```python
from build123d import *

# Parameters (mm, degrees)
BOSS_EXTRUDE1_DEPTH = 244.475
SKETCH2_R           = 3.429
CUT_EXTRUDE1_DEPTH  = 3.175
SKETCH3_R           = 3.429
CUT_EXTRUDE2_DEPTH  = 3.175


with BuildPart() as part:
    # Sketch1 → Boss-Extrude1 (new body)
    with BuildSketch(Plane(origin=(0, 0, 0), x_dir=(0, 0, -1), z_dir=(1, 0, 0))):
        Polygon((0, 0), (25.4, 0), (25.4, -3.175), (3.175, -3.175), (3.175, -25.4), (0, -25.4), align=None)
    extrude(amount=BOSS_EXTRUDE1_DEPTH)

    # Sketch2 → Cut-Extrude1 (cut)
    with BuildSketch(Plane.XY):
        with Locations((11.1125, -12.7)):
            Circle(SKETCH2_R)
        with Locations((36.5125, -12.7)):
            Circle(SKETCH2_R)
        with Locations((61.9125, -12.7)):
            Circle(SKETCH2_R)
        with Locations((182.5625, -12.7)):
            Circle(SKETCH2_R)
        with Locations((207.9625, -12.7)):
            Circle(SKETCH2_R)
        with Locations((233.3625, -12.7)):
            Circle(SKETCH2_R)
    extrude(amount=-CUT_EXTRUDE1_DEPTH, mode=Mode.SUBTRACT)

    # Sketch3 → Cut-Extrude2 (cut)
    with BuildSketch(Plane(origin=(0, 0, 0), x_dir=(1, 0, 0), z_dir=(0, 1, 0))):
        with Locations((11.8999, 19.05)):
            Circle(SKETCH3_R)
        with Locations((24.5999, 19.05)):
            Circle(SKETCH3_R)
        with Locations((37.2999, 19.05)):
            Circle(SKETCH3_R)
        with Locations((207.1751, 19.05)):
            Circle(SKETCH3_R)
        with Locations((219.8751, 19.05)):
            Circle(SKETCH3_R)
        with Locations((232.5751, 19.05)):
            Circle(SKETCH3_R)
    extrude(amount=-CUT_EXTRUDE2_DEPTH, mode=Mode.SUBTRACT)


solid = part.part
```
Build history of the part. All positions in model axes, mm. A direction names the side the tool comes from. Coordinates: 2 decimals unless noted, no trailing zeros. Order: outer loops, then holes, each group sorted by start corner. A loop starts at its lowest first (then second) coordinate and runs counter-clockwise, first axis right, second up. Notation, with made-up numbers: M 75.25,77.25 L 114.25,77.25 A13 ccw 114.25,81.25 Z; hole C -12,-14 d10. An arc over 180 degrees is marked long. One line per question, with ' | ' between items. Start each with the question number.
1. Mould opens along Z. For faces 1 (the face through (121, -13, 0)), 2 (the face through (14.28, -14.01, -1.57)), 3 (the face through (40.47, -1.57, -17.74)) say: +Z half, -Z half, draft (parallel to the pull), parting line (faces both ways), or undercut.
2. Wall check: line 1 along Z through (x, y) = (133, -14.75) (3 decimals). Give the ranges that are in metal, low to high. Write a range as [from, to].
3. Tool access for faces 4 (the face through (121, -3.175, -14)), 5 (the face through (0, -2, -8)): list every direction of +Z, -Z, +X, -X, +Y, -Y with a clear straight run to the whole face (end or side of a thin tool).
4. Cut at A-A (y = -12.7). Write the cut outline in (x, z) (1 decimal), plus the area to 3 significant figures.
5. Cut at D-D (z = -10.25). Write the cut outline in (x, y) (3 decimals).
6. Cut at B-B (z = -19.05). Write the cut outline in (x, y) (3 decimals), plus the area to 3 significant figures.
7. Cut at C-C (x = 112.5). Write the cut outline in (y, z) (3 decimals).
8. Flat gauge pins, fed straight in: P1, Ø10, axis at x = 51, y = -8.5, coming from the -Z side (3 decimals); P2, Ø8, axis at x = 232.58, z = -19.05, coming from the -Y side (3 decimals); P3, Ø4, axis at x = 61.91, y = -12.7, coming from the +Z side. Where does each tip first touch, or does it go through?
The answers:
1) face 1: +Z half | face 2: draft | face 3: undercut
2) line 1: z = [-3.175, 0]
3) face 4: -Z, +X, -X, -Y | face 5: +Z, -Z, -X, +Y, -Y
4) outline: M 0,-3.2 L 7.7,-3.2 L 7.7,0 L 0,0 Z; M 14.5,-3.2 L 33.1,-3.2 L 33.1,0 L 14.5,0 Z; M 39.9,-3.2 L 58.5,-3.2 L 58.5,0 L 39.9,0 Z; M 65.3,-3.2 L 179.1,-3.2 L 179.1,0 L 65.3,0 Z; M 186,-3.2 L 204.5,-3.2 L 204.5,0 L 186,0 Z; M 211.4,-3.2 L 229.9,-3.2 L 229.9,0 L 211.4,0 Z; M 236.8,-3.2 L 244.5,-3.2 L 244.5,0 L 236.8,0 Z | area: 646 mm2
5) outline: M 0,-3.175 L 244.475,-3.175 L 244.475,0 L 0,0 Z
6) outline: M 0,-3.175 L 8.471,-3.175 L 8.471,0 L 0,0 Z; M 15.329,-3.175 L 21.171,-3.175 L 21.171,0 L 15.329,0 Z; M 28.029,-3.175 L 33.871,-3.175 L 33.871,0 L 28.029,0 Z; M 40.729,-3.175 L 203.746,-3.175 L 203.746,0 L 40.729,0 Z; M 210.604,-3.175 L 216.446,-3.175 L 216.446,0 L 210.604,0 Z; M 223.304,-3.175 L 229.146,-3.175 L 229.146,0 L 223.304,0 Z; M 236.004,-3.175 L 244.475,-3.175 L 244.475,0 L 236.004,0 Z | area: 646 mm2
7) outline: M -25.4,-3.175 L -3.175,-3.175 L -3.175,-25.4 L 0,-25.4 L 0,0 L -25.4,0 Z
8) P1: stops at z = -3.175 | P2: stops at y = -3.175 | P3: passes through
